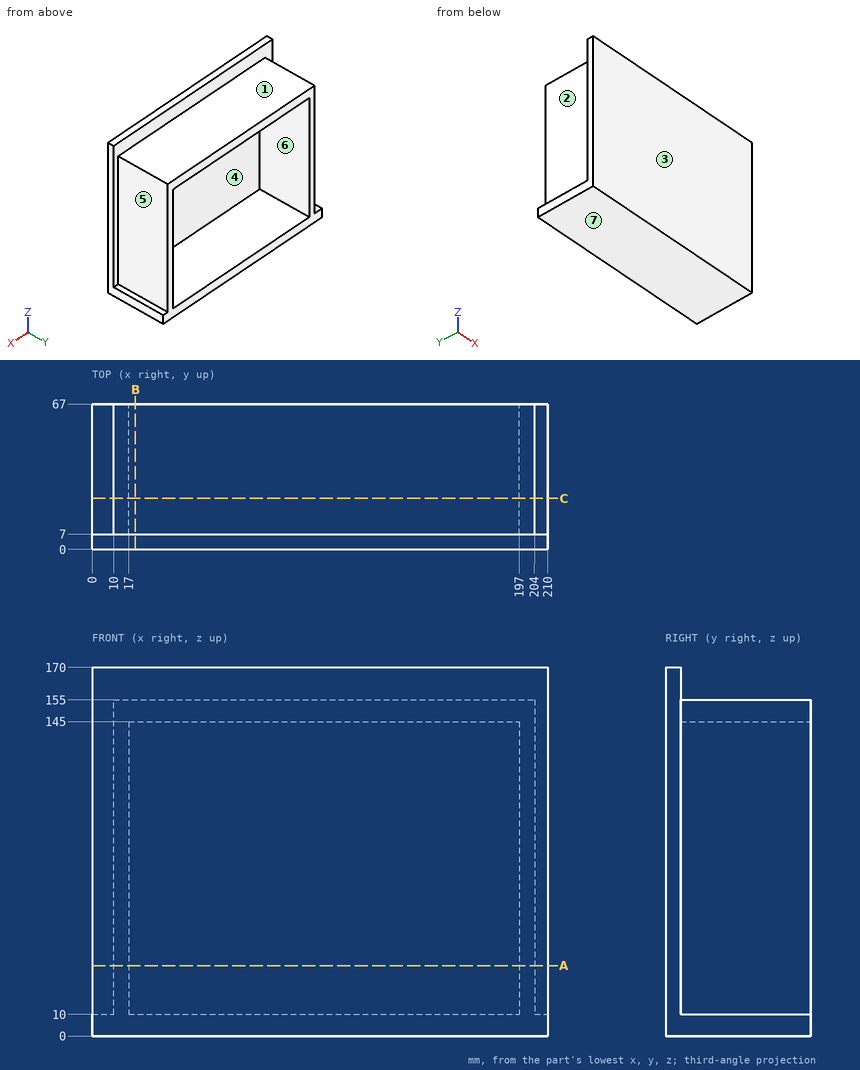
Check sheet for the drawn part. Datum: minimum x, y, z corner. Units: mm. A direction names the side the tool comes from. Round coordinates to 2 decimals unless told otherwise and drop trailing zeros. Order: outer loops, then holes, each group sorted by start corner. A loop starts at its lowest first (then second) coordinate and runs counter-clockwise, first axis right, second up. Notation, with made-up numbers: M 85,65.25 L 141,65.25 A21 cw 141,103.25 Z; hole C 72,-36 d4. An arc over 180 degrees is marked long. Write each question's results on one line, items separated by ' | '. Start each with the question number.
1. Material ranges on L1, parallel to Z at x = 150, y = 61; L2, parallel to X at y = 60, z = 91; L3, parallel to Y at x = 87.5, z = 114.5, recorded low to high. Write a range as from..to.
2. Set-up check for the marked faces 1, 2, 3 and 4: record each of +Z, -Z, +X, -X, +Y, -Y from which the full face is reachable in a straight line by a thin tool's end or side.
3. Cross-section at A-A on z = 32.5. Record the boundary of the cut face in (x, y), plus the area to 3 significant figures.
4. Draft check along Z on the marked faces 5, 6 and 7. Enter one of: pulls with the +Z half, pulls with the -Z half, needs draft (parallel to the pull), parting line crosses it, or undercut.
5. Cross-section at C-C on y = 23.5. Record the boundary of the cut face in (x, z), plus the area to 3 significant figures.
6. Go/stop test with flat-tipped pins: P1, Ø3, axis at x = 4, y = 32, coming from the +Z side; P2, Ø3, axis at x = 108, z = 123.5, coming from the +Y side; P3, Ø12, axis at x = 149, z = 107.5, coming from the -Y side; P4, Ø18, axis at x = 149, y = 39.5, coming from the +Z side. Record where each tip stops, or that it passes through.
7. Cross-section at B-B on x = 20. Record the boundary of the cut face in (y, z), plus the area to 3 significant figures.
Resolved:
1) L1: 0..10, 145..155 | L2: 10..17, 197..204 | L3: 0..7
2) face 1: +Z, +X, -X, +Y | face 2: +Z, -X, +Y | face 3: +Z, -Z, +X, -X, -Y | face 4: +Y
3) outline: M 0,0 L 210,0 L 210,7 L 204,7 L 204,67 L 197,67 L 197,7 L 17,7 L 17,67 L 10,67 L 10,7 L 0,7 Z | area: 2,310 mm2
4) face 5: needs draft | face 6: undercut | face 7: pulls with the -Z half
5) outline: M 0,0 L 210,0 L 210,10 L 204,10 L 204,155 L 10,155 L 10,10 L 0,10 Z; hole M 17,10 L 197,10 L 197,145 L 17,145 Z | area: 5,930 mm2
6) P1: z = 10 | P2: y = 7 | P3: y = 0 | P4: z = 155
7) outline: M 0,0 L 67,0 L 67,10 L 7,10 L 7,145 L 67,145 L 67,155 L 7,155 L 7,170 L 0,170 Z | area: 2,390 mm2
